Study the drawing (mm; zero at the part's minimum x, y, z) and answer. Round coordinates to 2 decimals unless told otherwise and drop trailing zeros. Loops run counter-clockwise (first coordinate to the right, second up) from the corner with the lowest first, then second, coordinate; pieces in that order, holes last. Notation, with made-up numbers: M 54.25,62.5 L 66.25,62.5 A7 cw 66.25,68.5 Z; hole C -39.75,85 d6. An arc over 180 degrees is marked long. Write each question's results on one line, items separated by ' | '.
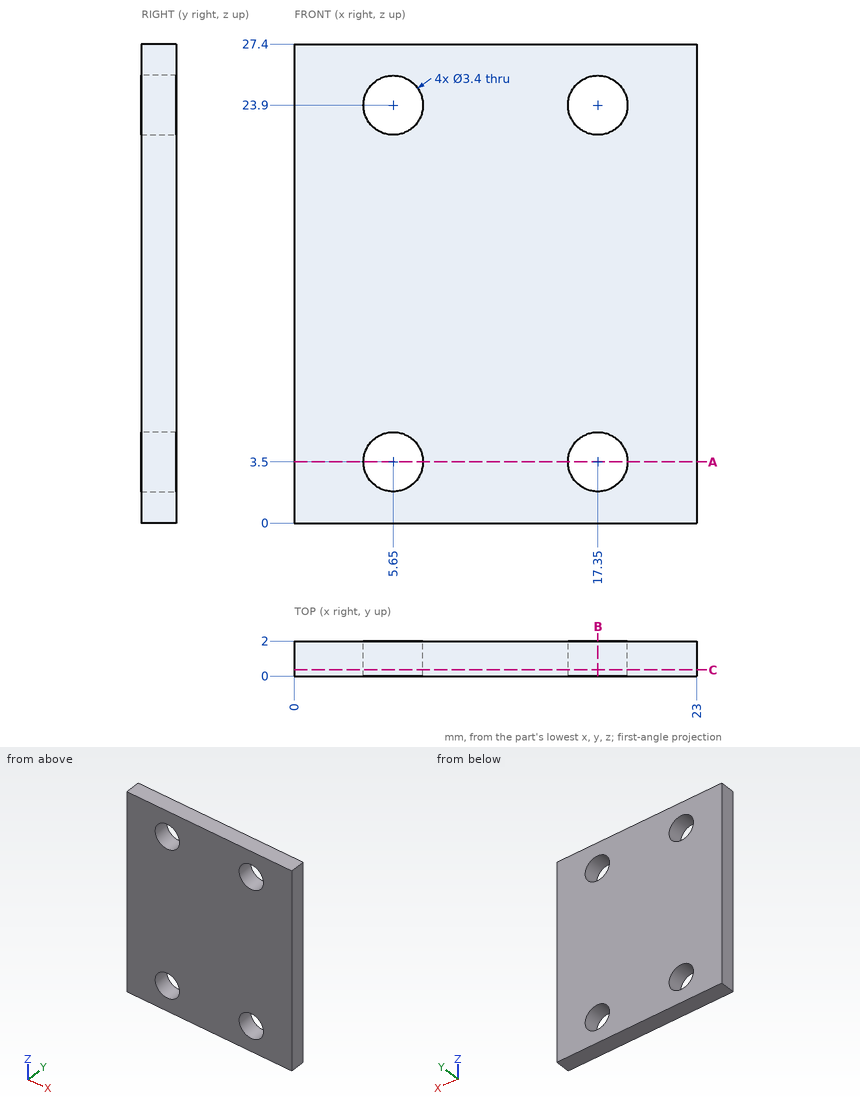
Item 1: The part is cut by section C-C (y = 0.35). Determine the outline of the cut face in (x, z).
Outcome:
outline: M 0,0 L 23,0 L 23,27.4 L 0,27.4 Z; hole C 5.65,3.5 d3.4; hole C 5.65,23.9 d3.4; hole C 17.35,3.5 d3.4; hole C 17.35,23.9 d3.4
Item 2: Straight lines are drawn through the part: line 1 (X direction, y = 0.5, z = 3.5); line 2 (Z direction, x = 17.5, y = 1.8); line 3 (X direction, y = 0.65, z = 4.25). For each, find the intervals that lie inside material, in ascending order.
Outcome:
line 1: x = 0 to 3.95, 7.35 to 15.65, 19.05 to 23 | line 2: z = 0 to 1.81, 5.19 to 22.21, 25.59 to 27.4 | line 3: x = 0 to 4.12, 7.18 to 15.82, 18.88 to 23
Item 3: The part is cut by section B-B (x = 17.35). Determine the outline of the cut face in (y, z).
Outcome:
outline: M 0,0 L 2,0 L 2,1.8 L 0,1.8 Z; M 0,5.2 L 2,5.2 L 2,22.2 L 0,22.2 Z; M 0,25.6 L 2,25.6 L 2,27.4 L 0,27.4 Z
Item 4: The part is cut by section A-A (z = 3.5). Determine the outline of the cut face in (x, y).
Outcome:
outline: M 0,0 L 3.95,0 L 3.95,2 L 0,2 Z; M 7.35,0 L 15.65,0 L 15.65,2 L 7.35,2 Z; M 19.05,0 L 23,0 L 23,2 L 19.05,2 Z
